Could you check a few things on this drawing? It's one solid part, dimensions in mm from its lowest x, y, z. Give positions to 0.01 mm unless a question says otherwise; leave off trailing zeros. Loops run counter-clockwise (first coordinate to the right, second up) from the corner with the lowest first, then second, coordinate; pieces in that order, holes last. Notation, with made-up numbers: (-39.75, 61) - (17.25, 61) arc R13 ccw to (17.25, 82) - close; hole circle Ø4 at (-39, -17.5). An arc over 180 degrees is marked (long way). Answer as a JSON object with one key per item and string values.
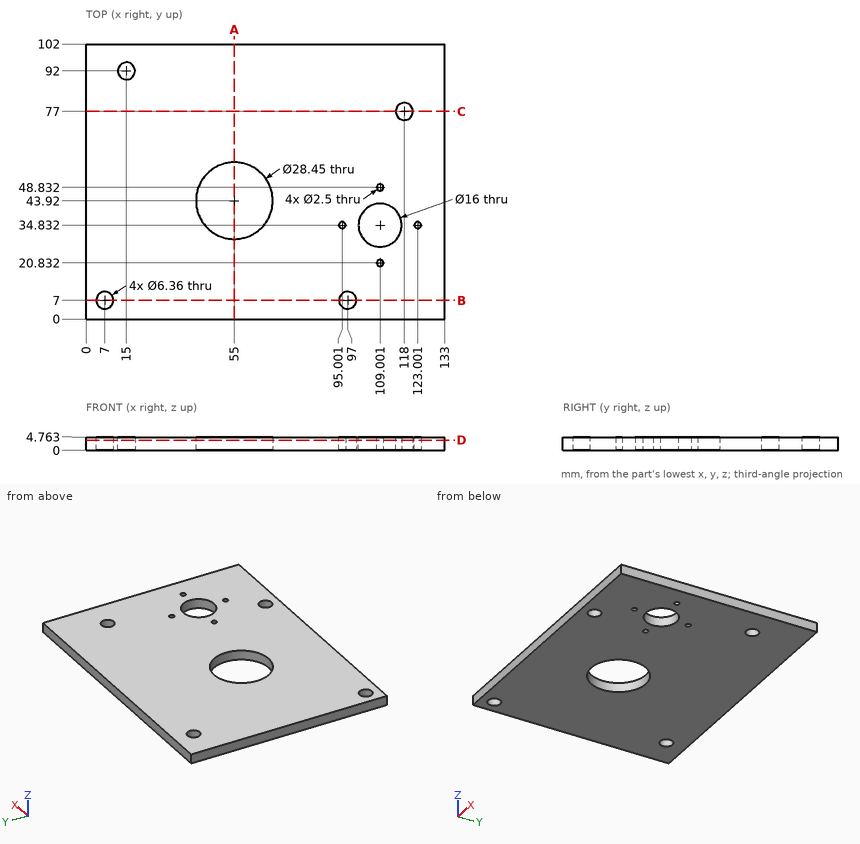
1) I need wall thicknesses on L1, parallel to Y at x = 7, z = 1.55; L2, parallel to Y at x = 108, z = 1.65 (1 decimal); L3, parallel to Y at x = 15, z = 1.1. Which ranges of each line are inside material? Lowest first, please.
Check sheet entries:
{"L1": "0 to 3.82, 10.18 to 102", "L2": "0 to 20.1, 21.6 to 26.9, 42.8 to 48.1, 49.6 to 102", "L3": "0 to 88.82, 95.18 to 102"}
2) I'm going to push a flat-ended pin straight in: P1, Ø5.5, axis at x = 7, y = 7, coming from the -Z side. Where does the tip first touch, or does it pass through?
Check sheet entries:
{"P1": "through"}
3) Imagine slicing it at B-B on y = 7. Write out the boundary of the cut face in (x, z).
Check sheet entries:
{"outline": "(0, 0) - (3.82, 0) - (3.82, 4.76) - (0, 4.76) - close; (10.18, 0) - (93.82, 0) - (93.82, 4.76) - (10.18, 4.76) - close; (100.18, 0) - (133, 0) - (133, 4.76) - (100.18, 4.76) - close"}
4) Imagine slicing it at A-A on x = 55. Write out the boundary of the cut face in (y, z) (1 decimal).
Check sheet entries:
{"outline": "(0, 0) - (29.7, 0) - (29.7, 4.8) - (0, 4.8) - close; (58.1, 0) - (102, 0) - (102, 4.8) - (58.1, 4.8) - close"}
5) Imagine slicing it at D-D on z = 3.65. Give the number of separate pieces and of enclosed holes in the cut face, and give its area (3 significant figures).
Check sheet entries:
{"separate pieces": "1", "enclosed holes": "10", "area": "12,600 mm2"}
6) Imagine slicing it at C-C on y = 77. Write out the boundary of the cut face in (x, z), and give its area (3 significant figures).
Check sheet entries:
{"outline": "(0, 0) - (114.82, 0) - (114.82, 4.76) - (0, 4.76) - close; (121.18, 0) - (133, 0) - (133, 4.76) - (121.18, 4.76) - close", "area": "603 mm2"}
